Read the model definition and answer for the solid it produces. Units are mm, in the model's axes. Face numbers are marked on the shaded views. A direction names the side the tool comes from. Coordinates: 2 decimals unless noted, no trailing zeros. Order: outer loops, then holes, each group sorted by start corner. A loop starts at its lowest first (then second) coordinate and runs counter-clockwise, first axis right, second up. Notation, with made-up numbers: M 17.5,6.25 L 61.5,6.25 A23 ccw 61.5,20.25 Z; hole C 56,-9.5 d11. An arc over 180 degrees is marked long. Write each question's results on one line, items separated by ' | '.
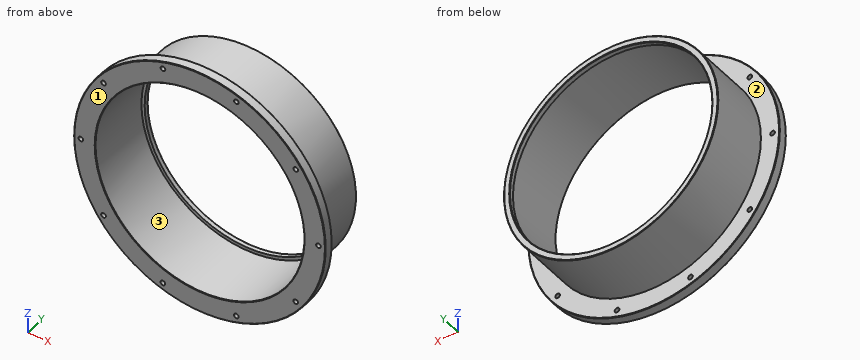
Autodesk Inventor part; units mm, degrees
ref_plane "YZ Plane" through (0, 0, 0) normal (1, 0, 0) x (0, 1, 0)
ref_plane "XZ Plane" through (0, 0, 0) normal (0, 1, 0) x (-1, 0, 0)
ref_plane "XY Plane" through (0, 0, 0) normal (0, 0, 1) x (1, 0, 0)
sketch "Sketch1" plane through (0, 0, 0) normal (0, 1, 0) x (-1, 0, 0)
  circle A0 centre (0, 0) radius 135
  circle A1 centre (0, 0) radius 115
  circle A2 centre (0, 0) radius 112.125
  circle A3 centre (0, 0) radius 9.5
  dimension "Absolute_Diameter" = 270
  dimension "Diameter_No_Outer_Lip" = 230
  dimension "Inner_Cylinder_Diameter" = 224.25
  dimension "Lip_Diameter" = 19
extrude "Extrusion1" add sketch "Sketch1" along normal blind 10 contours A0
extrude "Extrusion2" add sketch "Sketch1" along normal blind 75 contours A1
sketch "Sketch2" plane through (0, 75, 0) normal (0, 1, 0) x (1, 0, 0)
  circle A0 centre (0, 0) radius 115
  circle A1 centre (0, 0) radius 108.625
  dimension "Lip_Diameter_Out" = 230
  dimension "Inner_Lip_Diameter" = 217.25
extrude "Extrusion7" add sketch "Sketch2" against normal blind 5
chamfer "Chamfer1" distance 0.5 angle 45 2 edges at (115, 75, 0) (-108.625, 75, 0)
chamfer "Chamfer2" distance 0.5 angle 45 3 edges at (135, 10, 0) (135, 0, 0) (112.125, 0, 0)
sketch "Sketch3" plane through (0, 10, 0) normal (0, 1, 0) x (1, 0, 0)
  circle A0 centre (0, 0) radius 127.5
  circle A1 centre (-127.5, 0) radius 2.5
  circle A2 centre (-103.1497, -74.9426) radius 2.5
  circle A3 centre (-39.3997, -121.2597) radius 2.5
  circle A4 centre (39.3997, -121.2597) radius 2.5
  circle A5 centre (103.1497, -74.9426) radius 2.5
  circle A6 centre (127.5, 0) radius 2.5
  circle A7 centre (103.1497, 74.9426) radius 2.5
  circle A8 centre (39.3997, 121.2597) radius 2.5
  circle A9 centre (-39.3997, 121.2597) radius 2.5
  circle A10 centre (-103.1497, 74.9426) radius 2.5
  dimension "d27" = 255
  dimension "d28" = 5
  dimension "d31" = 360
extrude "Extrusion8" cut sketch "Sketch3" against normal blind 10 contours A0 A6 | A0 A6 | A7 A0 | A0 A7 | A5 A0 | A0 A5 | A8 A0 | A0 A8 | A4 A0 | A0 A4 | A9 A0 | A0 A9 | A3 A0 | A0 A3 | A10 A0 | A0 A10 | A2 A0 | A0 A2 | A1 A0 | A0 A1
sketch "Sketch4" plane through (0, 75, 0) normal (0, 1, 0) x (1, 0, 0)
  circle A0 centre (0, 0) radius 42.5
  circle A1 centre (0, 0) radius 37.5
  circle A2 centre (0, 0) radius 40
  circle A3 centre (-40, 0) radius 1
  circle A4 centre (-24.9396, -31.2733) radius 1
  circle A5 centre (8.9008, -38.9971) radius 1
  circle A6 centre (36.0388, -17.3553) radius 1
  circle A7 centre (36.0388, 17.3553) radius 1
  circle A8 centre (8.9008, 38.9971) radius 1
  circle A9 centre (-24.9396, 31.2733) radius 1
  dimension "d35" = 80
  dimension "d36" = 2
  dimension "d39" = 360
hole "Hole1" [suppressed]
properties part number "Cylinder  Segment - 01"
(1) The part is cut by section A-A, the plane y = 47. Write down the section's boundary in (x, z) (3 decimals).
Conclusion:
outline: C 0,0 d230; hole C 0,0 d224.25
(2) Given pin 1 (6.5 mm diameter, centred on x = 39.4, z = 121.26, fed in from +Y); pin 2 (8 mm diameter, centred on y = 43, z = 14, fed in from +X); pin 3 (8 mm diameter, centred on y = 23.5, z = -86.5, fed in from +X), each flat-ended and moving along its own axis, determine where each tip first touches the part or whether it passes through.
Conclusion:
pin 1: y = 10 | pin 2: x = 114.56 | pin 3: x = 80.12
(3) For the marked faces 1, 2 and 3, determine the directions among +Z, -Z, +X, -X, +Y, -Y from which every point of the face is accessible in a straight line to the end or side of a thin tool.
Conclusion:
face 1: +Z, -Z, +X, -X, -Y | face 2: +Y | face 3: -Y
(4) Straight lines are drawn through the part: line 1 (Z direction, x = 0, y = 73.4) (3 decimals); line 2 (Y direction, x = 120.5, z = -16); line 3 (X direction, y = 63.5, z = 59). For each, find the intervals that lie inside material, in ascending order.
Conclusion:
line 1: -115 to -108.625, 108.625 to 115 | line 2: 0 to 10 | line 3: -98.71 to -95.35, 95.35 to 98.71
